from build123d import *

# Parameters (mm, degrees)
SKETCH1_W           = 53.34
SKETCH1_H           = 158.75
SKETCH1_R           = 1.5875
BOSS_EXTRUDE1_DEPTH = 6.35
SKETCH2_3_W         = 32.258
SKETCH2_3_H         = 6.35
CUT_EXTRUDE2_DEPTH  = 137.662311459
SKETCH6_W           = 53.34
SKETCH6_H           = 6.35
BOSS_EXTRUDE5_DEPTH = 31.75
CUT_EXTRUDE3_REACH  = 165.072


with BuildPart() as part:
    # Sketch1 → Boss-Extrude1 (new body)
    with BuildSketch(Plane.XY):
        with Locations((-17.091445783, 49.935481928)):
            Rectangle(SKETCH1_W, SKETCH1_H)
        with Locations((-36.141445783, 69.620481928)):
            Circle(SKETCH1_R, mode=Mode.SUBTRACT)
        with Locations((-8.201445783, 69.620481928)):
            Circle(SKETCH1_R, mode=Mode.SUBTRACT)
        with Locations((-41.221445783, 121.690481928)):
            Circle(SKETCH1_R, mode=Mode.SUBTRACT)
        with Locations((7.038554217, 120.420481928)):
            Circle(SKETCH1_R, mode=Mode.SUBTRACT)
    extrude(amount=BOSS_EXTRUDE1_DEPTH)

    # Sketch2<3> → Cut-Extrude2 (cut, through all)
    with BuildSketch(Plane.XY.offset(6.35)):
        with Locations((-17.091445783, 60.014063864)):
            Rectangle(SKETCH2_3_W, SKETCH2_3_H)
    extrude(amount=-CUT_EXTRUDE2_DEPTH, mode=Mode.SUBTRACT)

    # Sketch6 → Boss-Extrude5 (add)
    with BuildSketch(Plane.XY.offset(6.35)):
        with Locations((-17.091445783, -26.264518072)):
            Rectangle(SKETCH6_W, SKETCH6_H)
    extrude(amount=BOSS_EXTRUDE5_DEPTH)

    # Sketch7 → Cut-Extrude3 (cut, up to next)
    with BuildSketch(Plane(origin=(0, -23.089518072, 0), x_dir=(1, 0, 0), z_dir=(0, 1, 0)), mode=Mode.PRIVATE) as cut_extrude3_sk1:
        with BuildLine():
            Line((-36.395445783, -21.844), (2.212554217, -21.844))
            ThreePointArc((2.212554217, -21.844), (5.768554217, -25.4), (2.212554217, -28.956))
            Line((2.212554217, -28.956), (-36.395445783, -28.956))
            ThreePointArc((-36.395445783, -28.956), (-39.951445783, -25.4), (-36.395445783, -21.844))
        make_face()
    cut_extrude3_tool1 = extrude(cut_extrude3_sk1.sketch, amount=-CUT_EXTRUDE3_REACH, mode=Mode.PRIVATE) & part.part
    add(cut_extrude3_tool1.solids().sort_by_distance((-17.091446, -23.089518, 25.4))[0], mode=Mode.SUBTRACT)


solid = part.part
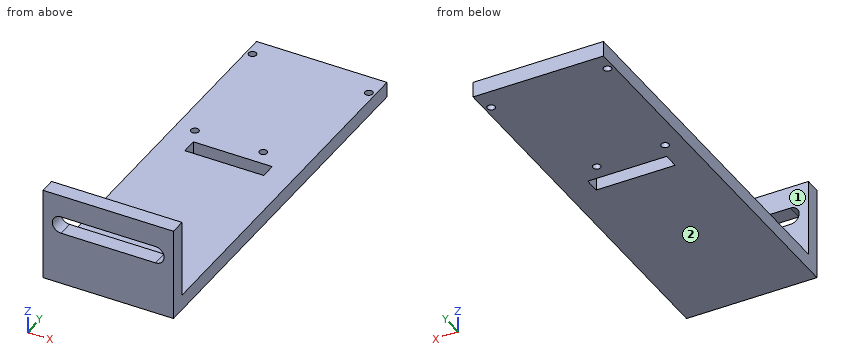
Here's how the part is built. I have some questions about the finished solid (model axes, mm). Face numbers are marked on the shaded views. A direction names the side the tool comes from. Give positions to 0.01 mm unless a question says otherwise; leave off trailing zeros. Write each loop counter-clockwise with the first axis right and the second up, starting at its lowest first coordinate (ties: lowest second). Pieces come first, ordered by that corner, then holes. Notation, with made-up numbers: (53.25, 59.5) -> (104.25, 59.5) arc R26 ccw to (104.25, 83.5) -> close; hole circle Ø9 at (77, 57). An arc over 180 degrees is marked (long way). Use one line per item in the form item = value. Start each with the question number.
1. On a 3-axis mill with a long thin cutter (end or side, diameter ignored), from which of +Z, -Z, +X, -X, +Y, -Y can I reach the whole of each face in a straight line? I mean the marked faces 1 and 2. Say none if no direction works.
2. Imagine slicing it at B-B on x = -20. List the corners of the cut face in (y, z) for me, plus the area to 3 significant figures.
3. Imagine slicing it at C-C on y = 9. List the corners of the cut face in (x, z) for me, plus the area to 3 significant figures.
4. If I drill on L1, parallel to Z at x = -1, y = 109; L2, parallel to Y at x = -6, z = 7.5, over which ranges is the centre line in solid material (lowest first)?
5. Imagine slicing it at A-A on z = 25.4. List the corners of the cut face in (x, y) for me.
6. Imagine slicing it at D-D on z = 11.5. List the corners of the cut face in (x, y) for me.
7. Will these pins go through, and if not, where does the flat tip stop? pin 1 Ø10 at (x, y) = (-33, -6.5) entering from +Z; pin 2 Ø12 at (x, z) = (-1.5, 15.5) entering from +Y.
Entries:
q1.face_1 = +Z, +X, -X, +Y
q1.face_2 = -Z, +X, -X, +Y, -Y
q2.outline = (-29.44, 0) -> (56.84, 0) -> (56.84, 6.35) -> (-23.09, 6.35) -> (-23.09, 21.84) -> (-29.44, 21.84) -> close; (-29.44, 28.96) -> (-23.09, 28.96) -> (-23.09, 38.1) -> (-29.44, 38.1) -> close; (63.19, 0) -> (129.31, 0) -> (129.31, 6.35) -> (63.19, 6.35) -> close
q2.area = 1,120 mm²
q3.outline = (-43.76, 0) -> (9.58, 0) -> (9.58, 6.35) -> (-43.76, 6.35) -> close
q3.area = 339 mm²
q4.L1 = 0 to 6.35
q4.L2 = -29.44 to -23.09
q5.outline = (-43.76, -29.44) -> (-39.95, -29.44) -> (-39.95, -23.09) -> (-43.76, -23.09) -> close; (5.77, -29.44) -> (9.58, -29.44) -> (9.58, -23.09) -> (5.77, -23.09) -> close
q6.outline = (-43.76, -29.44) -> (9.58, -29.44) -> (9.58, -23.09) -> (-43.76, -23.09) -> close
q7.pin_1 = 6.35
q7.pin_2 = -23.09
